For this review, take the finished solid that the model builds, in its own axes (mm). A direction names the side the tool comes from. Round coordinates to 2 decimals unless told otherwise and drop trailing zeros. Order: outer loops, then holes, each group sorted by start corner. A loop starts at its lowest first (then second) coordinate and runs counter-clockwise, first axis right, second up. Notation, with made-up numbers: M 29.5,59 L 51.5,59 A21 ccw 51.5,88 Z; hole C 9.25,31.25 d7. An arc over 180 degrees is marked long. Use a Markdown table: item, result.
from build123d import *

# Parameters (mm, degrees)
SALIENTE_EXTRUIR1_DEPTH    = 30
CORTAR_EXTRUIR2_DEPTH      = 42.46352267
CORTAR_EXTRUIR2_DEPTH_BACK = 42.46352267
CROQUIS3_W                 = 20
CROQUIS3_H                 = 40.792863267
CORTAR_EXTRUIR3_DEPTH      = 55.00268459
CORTAR_EXTRUIR3_DEPTH_BACK = 10
CROQUIS4_R                 = 1.5


with BuildPart() as part:
    # Croquis1 → Saliente-Extruir1 (new body)
    with BuildSketch(Plane.XY):
        with BuildLine():
            Line((-6.5, 20.93890902), (-6.5, 16.140322178))
            ThreePointArc((-6.5, 16.140322178), (0, -17.4), (6.5, 16.140322178))
            Line((6.5, 16.140322178), (6.5, 20.905653754))
            Line((6.5, 20.905653754), (11.5, 20.892863267))
            Line((11.5, 20.892863267), (11.5, 15.748015748))
            ThreePointArc((11.5, 15.748015748), (0, -19.5), (-11.5, 15.748015748))
            Line((-11.5, 15.748015748), (-11.5, 20.951699507))
            Line((-11.5, 20.951699507), (-6.5, 20.93890902))
        make_face()
    extrude(amount=SALIENTE_EXTRUIR1_DEPTH)

    # Croquis3 → Cortar-Extruir2 (cut, two sides: drawn at the far end of the back side and taken through both)
    with BuildSketch(Plane(origin=(0, 0, 0), x_dir=(0, 0, -1), z_dir=(1, 0, 0)).offset(-CORTAR_EXTRUIR2_DEPTH_BACK)):
        with Locations((-15, -2.003568366)):
            Rectangle(CROQUIS3_W, CROQUIS3_H)
    extrude(amount=CORTAR_EXTRUIR2_DEPTH + CORTAR_EXTRUIR2_DEPTH_BACK, mode=Mode.SUBTRACT)

    # Croquis4 → Cortar-Extruir3 (cut, two sides: drawn at the far end of the back side and taken through both)
    with BuildSketch(Plane(origin=(0.053520884, 20.922144475, 0), x_dir=(0.9999967280848749, -0.0025580890416273647, 0), z_dir=(0.0025580890416273647, 0.9999967280848749, 0)).offset(-CORTAR_EXTRUIR3_DEPTH_BACK)):
        with Locations((9, -2.5)):
            Circle(CROQUIS4_R)
        with Locations((-9, -2.5)):
            Circle(CROQUIS4_R)
        with Locations((-9, -27.5)):
            Circle(CROQUIS4_R)
        with Locations((9, -27.5)):
            Circle(CROQUIS4_R)
    extrude(amount=CORTAR_EXTRUIR3_DEPTH + CORTAR_EXTRUIR3_DEPTH_BACK, mode=Mode.SUBTRACT)


solid = part.part
Q1. Wall thickness on line 1 along X through (y, z) = (0, 27.5); line 2 along Z through (x, y) = (11.5, 15); line 3 along X through (y, z) = (-10.5, 4): over which ranges is each line inside the solid? List them lowest first. Write a range as [from, to].
Determined:
| item | result |
|---|---|
| line 1 | x = [-19.5, -17.4], [17.4, 19.5] |
| line 2 | z = [0, 5], [25, 30] |
| line 3 | x = [-16.43, -13.87], [13.87, 16.43] |
Q2. Add section A-A (z = 19.5). Write out the cut boundary in (x, y).
Determined:
| item | result |
|---|---|
| outline | M -11.5,18.39 L -6.5,18.39 L -6.5,20.94 L -11.5,20.95 Z; M 6.5,18.39 L 11.5,18.39 L 11.5,20.89 L 6.5,20.91 Z |
Q3. Add section B-B (y = -4.5). Write out the cut boundary in (x, z), then the cut area to 3 significant figures.
Determined:
| item | result |
|---|---|
| outline | M -18.97,0 L -16.81,0 L -16.81,5 L -18.97,5 Z; M -18.97,25 L -16.81,25 L -16.81,30 L -18.97,30 Z; M 16.81,0 L 18.97,0 L 18.97,5 L 16.81,5 Z; M 16.81,25 L 18.97,25 L 18.97,30 L 16.81,30 Z |
| area | 43.3 mm^2 |
Q4. Clearance check with flat-ended pins moving along their axes: pin 1 (5.5 mm diameter, centred on y = 18.5, z = 9.5, fed in from +X); pin 2 (1.4 mm diameter, centred on y = 19.5, z = 22, fed in from -X); pin 3 (5.5 mm diameter, centred on x = -8.5, z = 12, fed in from -Y); pin 4 (2 mm diameter, centred on x = 13.5, y = -10, fed in from +Z). State where each tip first meets the part, or that it passes through.
Determined:
| item | result |
|---|---|
| pin 1 | stops at x = 11.5 |
| pin 2 | stops at x = -11.5 |
| pin 3 | stops at y = 18.39 |
| pin 4 | stops at z = 30 |
Q5. Draft analysis for pull direction X (two halves, no side actions). For faces 4 (the cylindrical face through (-0.672, -17.387, 27.465)), 5 (the flat face through (1.4, -17.5, 25)), 6 (the flat face through (-11.5, 19, 15)), state which applies: pulls with the +X half, pulls with the -X half, needs draft (parallel to the pull), parting line crosses it, or undercut.
Determined:
| item | result |
|---|---|
| face 4 | undercut |
| face 5 | needs draft |
| face 6 | pulls with the -X half |
Q6. Machinability: for faces 1 (the flat face through (1.4, -17.5, 5)), 2 (the flat face through (-6.5, 19, 15)), 3 (the flat face through (11.5, 19, 15)), which of the approach directions +Z, -Z, +X, -X, +Y, -Y give a long, thin tool a straight path to every point of the face, cutting with its end or side? Answer none if there is none.
Determined:
| item | result |
|---|---|
| face 1 | +X, -X, -Y |
| face 2 | +Z, -Z, +Y |
| face 3 | +Z, -Z, +X, +Y |
Q7. Add section D-D (x = -14.5). Write out the cut boundary in (y, z), then the cut area to 3 significant figures.
Determined:
| item | result |
|---|---|
| outline | M -13.04,0 L -9.62,0 L -9.62,5 L -13.04,5 Z; M -13.04,25 L -9.62,25 L -9.62,30 L -13.04,30 Z; M 9.62,0 L 13.04,0 L 13.04,5 L 9.62,5 Z; M 9.62,25 L 13.04,25 L 13.04,30 L 9.62,30 Z |
| area | 68.4 mm^2 |
Q8. Add section C-C (x = 0). Write out the cut boundary in (y, z), then the cut area to 3 significant figures.
Determined:
| item | result |
|---|---|
| outline | M -19.5,0 L -17.4,0 L -17.4,5 L -19.5,5 Z; M -19.5,25 L -17.4,25 L -17.4,30 L -19.5,30 Z |
| area | 21.0 mm^2 |
